Can you work these out from the model? Positions are in its coordinate system, mm. Give positions to 0.01 mm unless a question says otherwise; leave off trailing zeros. Loops run counter-clockwise (first coordinate to the right, second up) from the corner with the lowest first, then second, coordinate; pieces in that order, holes last. Notation, with made-up numbers: (27.25, -20) -> (69.25, -20) arc R23 ccw to (69.25, -4) -> close; hole circle Ø5 at (-5, 16.5). An arc over 180 degrees is marked (long way). Return JSON: item names as keys, results as strings. Group by question number.
Q1. Suppose I cut it at A-A, the plane z = 4.5. Please give me the cut outline in (x, y).
Q2. I need wall thicknesses on line 1 along X through (y, z) = (22.75, 7.5); line 2 along X through (y, z) = (20.75, 10.25); line 3 along Y through (x, z) = (-45, 10.25). Which ranges of each line are inside material? Lowest first, please. Write a range as [from, to].
Q3. Suppose I cut it at D-D, the plane y = 18. Please give me the cut outline in (x, z).
Q4. Thinking about a two-plate mould opening in X: for faces 1 (the cylindrical face through (-134.436, 14.79, 5.193)), 2 (the flat face through (60, 15, 7)), 3 (the flat face through (-150, 15, 7)), 4 (the cylindrical face through (49.216, 14.79, 4.812)), which applies, pulls with the +X half, pulls with the -X half, needs draft (parallel to the pull), parting line crosses it, or undercut?
Q5. Suppose I cut it at C-C, the plane x = -130. Please give me the cut outline in (y, z).
Q6. Suppose I cut it at B-B, the plane y = 10. Please give me the cut outline in (x, z).
```python
from build123d import *

# Parameters (mm, degrees)
RESSALTO_EXTRUS_O1_DEPTH = 15
CORTE_EXTRUS_O1_DEPTH    = 15
ESBO_O3_R                = 5
CORTE_EXTRUS_O2_DEPTH    = 30


with BuildPart() as part:
    # Esboço1 → Ressalto-extrusão1 (new body)
    with BuildSketch(Plane.XY):
        Polygon((0, 0), (60, 0), (60, 30), (-150, 30), (-150, 0), align=None)
    extrude(amount=RESSALTO_EXTRUS_O1_DEPTH)

    # Esboço2 → Corte-extrusão1 (cut)
    with BuildSketch(Plane.XY.offset(15)):
        with BuildLine():
            ThreePointArc((-45, 22.5), (-52.5, 15), (-45, 7.5))
            Line((-45, 7.5), (-45, 22.5))
        make_face()
        with BuildLine():
            Line((-45, 22.5), (-45, 7.5))
            ThreePointArc((-45, 7.5), (-39.696699141, 9.696699141), (-37.5, 15))
            ThreePointArc((-37.5, 15), (-39.696699141, 20.303300859), (-45, 22.5))
        make_face()
    extrude(amount=-CORTE_EXTRUS_O1_DEPTH, mode=Mode.SUBTRACT)

    # Esboço3 → Corte-extrusão2 (cut)
    with BuildSketch(Plane(origin=(0, 0, 0), x_dir=(-1, 0, 0), z_dir=(0, -1, 0))):
        with Locations(Location((130, -7.5, 0), (0, 0, 90))):
            Circle(ESBO_O3_R)
        with Locations(Location((-45, -7.5, 0), (0, 0, 90))):
            Circle(ESBO_O3_R)
    extrude(amount=-CORTE_EXTRUS_O2_DEPTH, mode=Mode.SUBTRACT)


solid = part.part
```
Ans:
{
 "1": {"outline": "(-150, 0) -> (-134, 0) -> (-134, 30) -> (-150, 30) -> close; (-126, 0) -> (41, 0) -> (41, 30) -> (-126, 30) -> close; (49, 0) -> (60, 0) -> (60, 30) -> (49, 30) -> close; hole circle Ø15 at (-45, 15)"},
 "2": {"line 1": "x = [-150, -135], [-125, 40], [50, 60]", "line 2": "x = [-150, -134.18], [-125.82, -49.82], [-40.18, 40.82], [49.18, 60]", "line 3": "y = [0, 7.5], [22.5, 30]"},
 "3": {"outline": "(-150, 0) -> (-51.87, 0) -> (-51.87, 15) -> (-150, 15) -> close; (-38.13, 0) -> (60, 0) -> (60, 15) -> (-38.13, 15) -> close; hole circle Ø10 at (-130, 7.5); hole circle Ø10 at (45, 7.5)"},
 "4": {"face 1": "undercut", "face 2": "pulls with the +X half", "face 3": "pulls with the -X half", "face 4": "undercut"},
 "5": {"outline": "(0, 0) -> (30, 0) -> (30, 2.5) -> (0, 2.5) -> close; (0, 12.5) -> (30, 12.5) -> (30, 15) -> (0, 15) -> close"},
 "6": {"outline": "(-150, 0) -> (-50.59, 0) -> (-50.59, 15) -> (-150, 15) -> close; (-39.41, 0) -> (60, 0) -> (60, 15) -> (-39.41, 15) -> close; hole circle Ø10 at (-130, 7.5); hole circle Ø10 at (45, 7.5)"}
}
